Check sheet for the modelled part. Datum: model origin and axes. Units: mm. Round coordinates to 2 decimals unless told otherwise and drop trailing zeros. Loops run counter-clockwise (first coordinate to the right, second up) from the corner with the lowest first, then second, coordinate; pieces in that order, holes last. Notation, with made-up numbers: (44.25, 62.5) - (98.25, 62.5) arc R8 cw to (98.25, 71.5) - close; hole circle Ø10 at (9.25, -7.75). An arc over 180 degrees is marked (long way). Put each result on its own line as item: value. Start each with the question number.
```python
from build123d import *

# Parameters (mm, degrees)
F1_DEPTH = 127


with BuildPart() as f1:
    # F0 (on Top) → F1 (new body)
    with BuildSketch(Plane.XY):
        with BuildLine():
            Line((-61.079588, 0), (0, 0))
            Line((0, 0), (-17.086972, 29.594812))
            Line((-17.086972, 29.594812), (-37.100383, 28.799639))
            ThreePointArc((-37.100383, 28.799639), (-37.020352, 28.013477), (-36.993634, 27.223703))
            ThreePointArc((-36.993634, 27.223703), (-49.006091, 15.542063), (-60.347805, 27.875973))
            Line((-60.347805, 27.875973), (-76.764559, 27.223703))
            Line((-76.764559, 27.223703), (-61.079588, 0))
        make_face()
    extrude(amount=F1_DEPTH)


solid = f1.part
```
Q1. Cross-section at A-A on z = 11. Enter the section's corners in (x, y).
Q2. Cross-section at C-C on x = -7. Enter the section's corners in (y, z), and give its area (3 significant figures).
Q3. Cross-section at D-D on y = 7.5. Enter the section's corners in (x, z).
Q4. Cross-section at B-B on y = 20. Enter the section's corners in (x, z), and give its area (3 significant figures).
Q5. Depth check by flat-ended pin: pin 1 Ø5 at (y, z) = (24.5, 108) entering from -X; pin 2 Ø4 at (y, z) = (22.5, 20) entering from +X; pin 3 Ø2 at (x, z) = (-44.5, 34) entering from +Y. Enter the tip coordinate at first touch or a pass-through.
Q6. Material ranges on line 1 (Y direction, x = -48, z = 75); line 2 (X direction, y = 21.25, z = 101); line 3 (X direction, y = 21.75, z = 11.5), recorded low to high. Write a range as from..to.
Q7. Draft check along X on faces 1 (the face through (-27, 29.2, 62.6)), 2 (the face through (-39, 12, 127)), 3 (the face through (-48.745, 15.538, 62.611)). Enter one of: +X half, -X half, draft (parallel to the pull), parting line (faces both ways), or undercut.
Answer list:
1. outline: (-76.76, 27.22) - (-61.08, 0) - (0, 0) - (-17.09, 29.59) - (-37.1, 28.8) arc R11.69 cw to (-36.99, 27.22) arc R11.69 cw (long way) to (-60.35, 27.88) - close
2. outline: (0, 0) - (12.12, 0) - (12.12, 127) - (0, 127) - close
2. area: 1,540 mm2
3. outline: (-65.4, 0) - (-4.33, 0) - (-4.33, 127) - (-65.4, 127) - close
4. outline: (-72.6, 0) - (-57.87, 0) - (-57.87, 127) - (-72.6, 127) - close; (-39.49, 0) - (-11.55, 0) - (-11.55, 127) - (-39.49, 127) - close
4. area: 5,420 mm2
5. pin 1: stops at x = -76.64
5. pin 2: stops at x = -11.84
5. pin 3: stops at y = 16.75
6. line 1: y = 0..15.56
6. line 2: x = -73.32..-58.72, -38.64..-12.27
6. line 3: x = -73.61..-59, -38.35..-12.56
7. face 1: -X half
7. face 2: draft
7. face 3: undercut
